Solid Edge part; units mm, degrees
sketch "Sketch1" plane through (0, 0, 0) normal (0, 0, 1) x (1, 0, 0)
  line L0 (-19.5, 20.7846) -> (-19.5, -20.7846)
  arc A0 (19.5, -20.7846) -> (-19.5, -20.7846) centre (0, 0) cw
  line L1 (19.5, -20.7846) -> (19.5, 20.7846)
  arc A1 (-19.5, 20.7846) -> (19.5, 20.7846) centre (0, 0) cw
extrude "Protrusion1" add sketch "Sketch1" against normal blind 23
shell "Thinwall1" thickness 0.85 removed faces 1 at (-13.39, -18.43, 0)
sketch "Sketch2" plane through (0, 0, -22.15) normal (0, 0, 1) x (0, 1, 0)
  line L0 (-16, -5) -> (-16, 5)
  line L1 (-8, 5) -> (-16, 5)
  line L2 (-8, -5) -> (-8, 5)
  line L3 (-8, -5) -> (-16, -5)
  line L4 (8, -5) -> (16, -5)
  line L5 (16, -5) -> (16, 5)
  line L6 (8, 5) -> (16, 5)
  line L7 (8, -5) -> (8, 5)
extrude "Cutout1" cut sketch "Sketch2" against normal blind 41.275
fillet "Round1" radius 1 4 edges at (19.5, -20.7846, -11.5) (19.5, 20.7846, -11.5) (-19.5, 20.7846, -11.5) (-19.5, -20.7846, -11.5)
fillet "Round2" radius 0.3 8 edges at (0, -28.5, 0) (19.4145, -20.7515, 0) (-19.4145, -20.7515, 0) (19.5, 0, 0) (-19.5, 0, 0) (19.4145, 20.7515, 0) (-19.4145, 20.7515, 0) (0, 28.5, 0)
fillet "Round3" radius 1 8 edges at (0, -28.5, -23) (19.4145, -20.7515, -23) (-19.4145, -20.7515, -23) (19.5, 0, -23) (-19.5, 0, -23) (19.4145, 20.7515, -23) (-19.4145, 20.7515, -23) (0, 28.5, -23)
properties material "boot"
Input: part model. Units: mm. Frame: model coordinates. A direction names the side the tool comes from. Coordinates: 2 decimals unless noted, no trailing zeros. Loops run counter-clockwise (first coordinate to the right, second up) from the corner with the lowest first, then second, coordinate; pieces in that order, holes last.
(1) Section A-A on z = -20. Return the cut outline in (x, y).
(2) Section B-B on y = 11. Return the cut outline in (x, z), then the cut area to 3 significant figures.
(3) First-contact query: pin 1 Ø12 at (x, z) = (13, -8.5) entering from +Y; pin 2 Ø8 at (x, z) = (14.5, -7.5) entering from -Y; pin 3 Ø0.7 at (x, z) = (2.5, -22.5) entering from +Y. Flat tips, straight axial feed; report the tip coordinate or a pass-through.
(4) Pull-direction query (Y, two-part tool) for faces 1 (the face through (19.5, 0, -11)), 2 (the face through (0, 0, -22.15)), 3 (the face through (-0.3, -28.5, -11)); classes: released by +Y, released by -Y, zero draft, split by the parting line, or undercut.
(5) Set-up query: faces 4 (the face through (-18.65, 0, -11)), 5 (the face through (0, 0, -23)). Return all of +Z, -Z, +X, -X, +Y, -Y with unobstructed straight access to the full face (end or side cutting, diameter ignored); none if empty.
(6) Section C-C on x = 2.5. Count the separate pieces of the cut face and the enclosed holes in it, then the cut area to 3 significant figures.
(7) Material intervals for probe 1 along X at (y, z) = (3, -7.25); probe 2 along Z at (x, y) = (-8, -12.5); probe 3 along Y at (x, z) = (10, -20), sorted ascending.
Data:
1. outline: (-19.5, -20.35) arc R1 ccw to (-19.17, -21.09) arc R28.5 ccw to (19.17, -21.09) arc R1 ccw to (19.5, -20.35) - (19.5, 20.35) arc R1 ccw to (19.17, 21.09) arc R28.5 ccw to (-19.17, 21.09) arc R1 ccw to (-19.5, 20.35) - close; hole (-18.65, -20.41) arc R27.65 ccw to (18.65, -20.41) - (18.65, 20.41) arc R27.65 ccw to (-18.65, 20.41) - close
2. outline: (-19.5, -22) arc R1 ccw to (-18.5, -23) - (-5, -23) - (-5, -22.15) - (-18.65, -22.15) - (-18.65, 0) - (-19.2, 0) arc R0.3 ccw to (-19.5, -0.3) - close; (5, -23) - (18.5, -23) arc R1 ccw to (19.5, -22) - (19.5, -0.3) arc R0.3 ccw to (19.2, 0) - (18.65, 0) - (18.65, -22.15) - (5, -22.15) - close
2. area: 61.8 mm2
3. pin 1: stops at y = 27.63
3. pin 2: stops at y = -26.5
3. pin 3: stops at y = 28.39
4. face 1: zero draft
4. face 2: undercut
4. face 3: released by -Y
5. face 4: +Z
5. face 5: -Z, +X, -X, +Y, -Y
6. separate pieces: 3
6. enclosed holes: 0
6. area: 72.0 mm2
7. probe 1: x = -19.5 to -18.65, 18.65 to 19.5
7. probe 2: z = -23 to -22.15
7. probe 3: y = -26.69 to -25.78, 25.78 to 26.69
